Can you work these out from the model? Positions are in its coordinate system, mm. Face numbers are marked on the shaded views. A direction names the side the tool comes from. Give positions to 0.01 mm unless a question says otherwise; leave off trailing zeros. Write each loop counter-clockwise with the first axis right and the second up, starting at its lowest first coordinate (ties: lowest second). Pieces come first, ordered by that corner, then holes. Notation, with made-up numbers: M -33,83 L -22,83 A30 ccw -22,119 Z; hole C -4.75,3 d4. An arc over 180 degrees is marked long. Write each question's results on one line, items separated by ' | '.
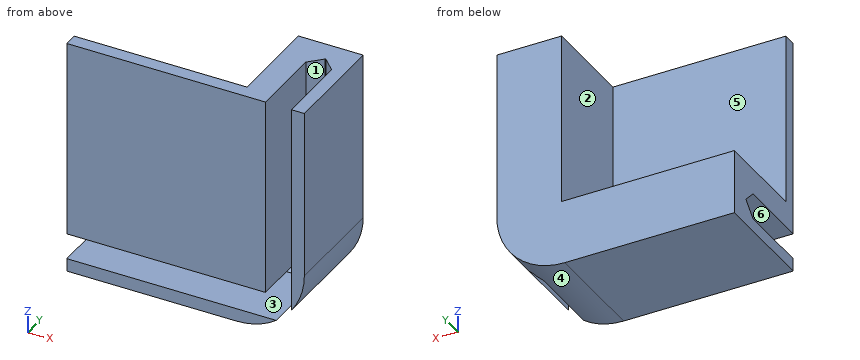
Autodesk Inventor part; units mm, degrees
ref_plane "YZ Plane" through (0, 0, 0) normal (1, 0, 0) x (0, 1, 0)
ref_plane "XZ Plane" through (0, 0, 0) normal (0, 1, 0) x (-1, 0, 0)
ref_plane "XY Plane" through (0, 0, 0) normal (0, 0, 1) x (1, 0, 0)
sketch "Sketch1" plane through (0, 0, 0) normal (0, 1, 0) x (-1, 0, 0)
  line L0 (0, 0) -> (-9.525, 0)
  line L1 (-9.525, 0) -> (-9.525, -9.525)
  line L2 (-9.525, -9.525) -> (0, -9.525)
  line L3 (0, -9.525) -> (0, 0)
  line L4 (0, 0) -> (25.4, 0)
  line L5 (25.4, 0) -> (25.4, -9.525)
  line L6 (25.4, -9.525) -> (0, -9.525)
  line L7 (0, -9.525) -> (0, 0)
  line L8 (0, 0) -> (-9.525, 0)
  line L9 (-9.525, 0) -> (-9.525, 25.4)
  line L10 (-9.525, 25.4) -> (0, 25.4)
  line L11 (0, 25.4) -> (0, 0)
  dimension "d0" = 9.525
  dimension "d1" = 9.525
  dimension "d2" = 25.4
  dimension "d3" = 9.525
  dimension "d4" = 9.525
  dimension "d5" = 25.4
extrude "Extrusion1" add sketch "Sketch1" along normal blind 15.875
sketch "Sketch2" plane through (0, 0, 0) normal (0, -1, 0) x (1, 0, 0)
  line L0 (0, 0) -> (7.62, 0) construction
  line L1 (7.62, 0) -> (7.62, -7.62) construction
  line L2 (7.62, -7.62) -> (0, -7.62) construction
  line L3 (0, -7.62) -> (0, 0) construction
  line L4 (7.62, -7.62) -> (3.81, -7.62)
  line L5 (3.81, -7.62) -> (3.81, 25.4)
  line L6 (3.81, 25.4) -> (7.62, 25.4)
  line L7 (7.62, 25.4) -> (7.62, -7.62)
  line L8 (7.62, -7.62) -> (-25.4, -7.62)
  line L9 (-25.4, -7.62) -> (-25.4, -3.81)
  line L10 (-25.4, -3.81) -> (7.62, -3.81)
  line L11 (7.62, -3.81) -> (7.62, -7.62)
  dimension "d8" = 7.62
  dimension "d9" = 7.62
  dimension "d10" = 3.81
  dimension "d11" = 33.02
  dimension "d12" = 33.02
  dimension "d13" = 3.81
extrude "Extrusion2" cut sketch "Sketch2" against normal blind 12.7
fillet "Fillet1" radius 10 1 edges at (9.525, 7.9375, -9.525)
chamfer "Chamfer1" distance 1.8415 angle 45 4 edges at (7.62, 12.7, 10.0019) (3.81, 12.7, 10.795) (-10.795, 12.7, -3.81) (-10.0019, 12.7, -7.62)
sketch "Sketch3" plane through (0, 0, 0) normal (0, -1, 0) x (1, 0, 0)
  line L0 (0, 0) -> (-25.4, 0)
  line L1 (-25.4, 0) -> (-25.4, 25.4)
  line L2 (-25.4, 25.4) -> (0, 25.4)
  line L3 (0, 25.4) -> (0, 0)
  dimension "d20" = 25.4
  dimension "d21" = 25.4
extrude "Extrusion3" add sketch "Sketch3" against normal blind 2
properties part number "Corner Piece"
Item 1: For the marked faces 1, 2 and 3, which set-ups out of +Z, -Z, +X, -X, +Y, -Y let a thin tool reach every point of the face, with its end or its side?
Geometry says:
face 1: +Z, -Y | face 2: +Z, -X, +Y | face 3: +X, -X, -Y
Item 2: If I drill on line 1 (Z direction, x = -6.5, y = 4.25) (3 decimals); line 2 (Z direction, x = -15.5, y = 1.25) (3 decimals); line 3 (X direction, y = 7.5, z = 18.5) (3 decimals), over which ranges is the centre line in solid material (lowest first)? Write a range as from..to.
Geometry says:
line 1: z = -9.525..-7.62, -3.81..0 | line 2: z = -9.525..-7.62, -3.81..25.4 | line 3: x = 0..3.81, 7.62..9.525
Item 3: I'm going to push flat-ended pins straight in: pin 1 (2 mm diameter, centred on x = 4.5, y = 5.5, fed in from +Z); pin 2 (7 mm diameter, centred on x = -9, y = 9, fed in from +Z). Where does each tip first touch, or does it pass through?
Geometry says:
pin 1: stops at z = 25.4 | pin 2: stops at z = 0
Item 4: I want a section at B-B, the plane y = 13.75. Please give me the cut outline in (x, z) (3 decimals), and give its area (3 significant figures).
Geometry says:
outline: M -25.4,-9.525 L -0.475,-9.525 A10 ccw 9.525,0.475 L 9.525,25.4 L 0,25.4 L 0,0 L -25.4,0 Z | area: 553 mm2
Item 5: I want a section at D-D, the plane y = 7.25. Please give me the cut outline in (x, z) (3 decimals).
Geometry says:
outline: M -25.4,-9.525 L -0.475,-9.525 A10 ccw 5.396,-7.62 L -25.4,-7.62 Z; M -25.4,-3.81 L 3.81,-3.81 L 3.81,25.4 L 0,25.4 L 0,0 L -25.4,0 Z; M 7.62,-5.396 A10 ccw 9.525,0.475 L 9.525,25.4 L 7.62,25.4 Z
Item 6: Thinking about a two-plate mould opening in Z: for the marked faces 4, 5 and 6, which applies, +Z half, -Z half, draft (parallel to the pull), parting line (faces both ways), or undercut?
Geometry says:
face 4: -Z half | face 5: draft | face 6: undercut
